```python
from build123d import *

# Parameters (mm, degrees)
BOSS_EXTRUDE1_DEPTH = 5
SKETCH2_W           = 12
SKETCH2_H           = 32
BOSS_EXTRUDE2_DEPTH = 6
CUT_EXTRUDE1_REACH  = 53.952
AGUJEROSMOTOR_R     = 1.5
FILLET1_R           = 2
SKETCH5_W           = 35
SKETCH5_H           = 5
BOSS_EXTRUDE3_DEPTH = 13
FILLET2_R           = 2
FILLET3_R           = 2
FILLET4_R           = 2
BOSS_EXTRUDE4_DEPTH = 3


with BuildPart() as part:
    # Sketch U → Boss-Extrude1 (new body)
    with BuildSketch(Plane(origin=(0, 0, 0), x_dir=(0, 0, -1), z_dir=(1, 0, 0))):
        with BuildLine():
            Line((0, 22), (0, 27))
            Line((0, 27), (-41, 27))
            ThreePointArc((-41, 27), (-42.414213562, 26.414213562), (-43, 25))
            Line((-43, 25), (-43, -3))
            ThreePointArc((-43, -3), (-42.414213562, -4.414213562), (-41, -5))
            Line((-41, -5), (0, -5))
            Line((0, -5), (0, 0))
            Line((0, 0), (-35, 0))
            ThreePointArc((-35, 0), (-36.414213562, 0.585786438), (-37, 2))
            Line((-37, 2), (-37, 20))
            ThreePointArc((-37, 20), (-36.414213562, 21.414213562), (-35, 22))
            Line((-35, 22), (0, 22))
        make_face()
    extrude(amount=-BOSS_EXTRUDE1_DEPTH)

    # Sketch2 → Boss-Extrude2 (add)
    with BuildSketch(Plane(origin=(0, 0, 0), x_dir=(0, 0, -1), z_dir=(1, 0, 0))):
        with Locations((-6, 11)):
            Rectangle(SKETCH2_W, SKETCH2_H)
    extrude(amount=BOSS_EXTRUDE2_DEPTH)

    # AgujerosMotor → Cut-Extrude1 (cut, up to next)
    with BuildSketch(Plane(origin=(6, 0, 0), x_dir=(0, 0, -1), z_dir=(1, 0, 0)), mode=Mode.PRIVATE) as cut_extrude1_sk1:
        with Locations((-5, 2)):
            Circle(AGUJEROSMOTOR_R)
    cut_extrude1_tool1 = extrude(cut_extrude1_sk1.sketch, amount=-CUT_EXTRUDE1_REACH, mode=Mode.PRIVATE) & part.part
    # AgujerosMotor → Cut-Extrude1 (cut, up to next)
    with BuildSketch(Plane(origin=(6, 0, 0), x_dir=(0, 0, -1), z_dir=(1, 0, 0)), mode=Mode.PRIVATE) as cut_extrude1_sk2:
        with Locations((-5, 20)):
            Circle(AGUJEROSMOTOR_R)
    cut_extrude1_tool2 = extrude(cut_extrude1_sk2.sketch, amount=-CUT_EXTRUDE1_REACH, mode=Mode.PRIVATE) & part.part
    add(cut_extrude1_tool1.solids().sort_by_distance((6, 2, 5))[0], mode=Mode.SUBTRACT)
    add(cut_extrude1_tool2.solids().sort_by_distance((6, 20, 5))[0], mode=Mode.SUBTRACT)

    # Fillet1
    fillet1_edges = [part.edges().sort_by_distance(p)[0] for p in [
        (6, 27, 6),
        (6, -5, 6),
    ]]
    fillet(fillet1_edges, radius=FILLET1_R)

    # Sketch5 → Boss-Extrude3 (add)
    with BuildSketch(Plane.ZY.offset(5)):
        with Locations((17.5, 24.5)):
            Rectangle(SKETCH5_W, SKETCH5_H)
    extrude(amount=BOSS_EXTRUDE3_DEPTH)

    # Fillet2
    fillet2_edges = [part.edges().sort_by_distance(p)[0] for p in [
        (-18, 24.5, 35),
    ]]
    fillet(fillet2_edges, radius=FILLET2_R)

    # Fillet3
    fillet3_edges = [part.edges().sort_by_distance(p)[0] for p in [
        (0, -5, 26.5),
        (0, -4.414213562, 42.414213562),
        (0, 11, 43),
        (0, 26.414213562, 42.414213562),
        (0, 27, 26.5),
        (-5, 26.414213562, 42.414213562),
        (-5, 11, 43),
        (-5, -4.414213562, 42.414213562),
        (-5, -5, 20.5),
        (6, 11, 12),
        (2, -5, 12),
        (2, 27, 12),
        (5.414213562, -4.414213562, 12),
        (5.414213562, 26.414213562, 12),
        (-5, 27, 38),
    ]]
    fillet(fillet3_edges, radius=FILLET3_R)

    # Fillet4
    fillet4_edges = [part.edges().sort_by_distance(p)[0] for p in [
        (-18, 27, 16.5),
        (-17.414213562, 27, 34.414213562),
        (-9.5, 27, 35),
    ]]
    fillet(fillet4_edges, radius=FILLET4_R)

    # Encastre → Boss-Extrude4 (add)
    with BuildSketch(Plane(origin=(0, 27, 0), x_dir=(1, 0, 0), z_dir=(0, 1, 0))):
        with BuildLine():
            Line((-5, -5), (-5, -25))
            ThreePointArc((-5, -25), (-9, -29), (-13, -25))
            Line((-13, -25), (-13, -5))
            ThreePointArc((-13, -5), (-9, -1), (-5, -5))
        make_face()
    extrude(amount=BOSS_EXTRUDE4_DEPTH)


solid = part.part
```
The model under review builds one solid part; all positions refer to its coordinate system, in mm. A direction names the side the tool comes from. Give positions to 0.01 mm unless a question says otherwise; leave off trailing zeros. Write each loop counter-clockwise with the first axis right and the second up, starting at its lowest first coordinate (ties: lowest second). Pieces come first, ordered by that corner, then holes. Notation, with made-up numbers: (72, 58) -> (100, 58) arc R17 ccw to (100, 63) -> close; hole circle Ø6 at (86, 1.5). An arc over 180 degrees is marked (long way). Answer in a Markdown table with one row per item.
1) Tool access review of faces 1 (the flat face through (0, 11, 6)), 2 (the cylindrical face through (-2.46, 0.57, 36.4)), 3 (the flat face through (-5, 28, 15)), 4 (the cylindrical face through (-9.41, 26.4, 34.43)): name each direction out of +Z, -Z, +X, -X, +Y, -Y from which nothing blocks a thin tool from reaching the whole face with its end or side.
Worked answers:
| item | result |
|---|---|
| face 1 | -Z, -X |
| face 2 | -Z, +X, -X |
| face 3 | +Z, -Z, +X, +Y |
| face 4 | +Z, -X, +Y |
2) Add section D-D on z = 23. State the section outline as (x, y) points, plus the area to 3 significant figures.
Worked answers:
| item | result |
|---|---|
| outline | (-18, 22) -> (0, 22) -> (0, 25) arc R2 ccw to (-2, 27) -> (-5, 27) -> (-5, 30) -> (-13, 30) -> (-13, 27) -> (-16, 27) arc R2 ccw to (-18, 25) -> close; (-5, -3) arc R2 ccw to (-3, -5) -> (-2, -5) arc R2 ccw to (0, -3) -> (0, 0) -> (-5, 0) -> close |
| area | 136 mm² |
3) Add section A-A on z = 32.5. State the section outline as (x, y) points, plus the area to 3 significant figures.
Worked answers:
| item | result |
|---|---|
| outline | (-18, 22) -> (0, 22) -> (0, 25) arc R2 ccw to (-2, 27) -> (-16, 27) arc R2 ccw to (-18, 25) -> close; (-5, -3) arc R2 ccw to (-3, -5) -> (-2, -5) arc R2 ccw to (0, -3) -> (0, 0) -> (-5, 0) -> close |
| area | 112 mm² |
4) For L1, parallel to Y at x = 2.6, z = 5; L2, parallel to Y at x = 4.55, z = 5; L3, parallel to Y at x = -9.5, z = 32.5, list the stretches that pass through material, from the lowest coordinate up. Write a range as [from, to].
Worked answers:
| item | result |
|---|---|
| L1 | [-5, 0.5], [3.5, 18.5], [21.5, 27] |
| L2 | [-4.92, 0.5], [3.5, 18.5], [21.5, 26.92] |
| L3 | [22, 27] |
5) Add section B-B on y = 16. State the section outline as (x, z) points.
Worked answers:
| item | result |
|---|---|
| outline | (-5, 37) -> (0, 37) -> (0, 41) arc R2 ccw to (-2, 43) -> (-3, 43) arc R2 ccw to (-5, 41) -> close; (0, 0) -> (6, 0) -> (6, 10) arc R2 ccw to (4, 12) -> (0, 12) -> close |
6) Add section C-C on x = -9. State the section outline as (y, z) points.
Worked answers:
| item | result |
|---|---|
| outline | (22, 0) -> (27, 0) -> (27, 1) -> (30, 1) -> (30, 29) -> (27, 29) -> (27, 33) arc R2 ccw to (25, 35) -> (22, 35) -> close |
7) Clearance check with flat-ended pins moving along their axes: P1, Ø3, axis at x = 3, y = 11.5, coming from the +Z side; P2, Ø14, axis at y = 10, z = 26.5, coming from the -X side; P3, Ø12, axis at y = 1.5, z = 29.5, coming from the +X side; P4, Ø4.5, axis at x = 2, y = 10, coming from the +Z side. State where each tip first meets the part, or that it passes through.
Worked answers:
| item | result |
|---|---|
| P1 | z = 12 |
| P2 | through |
| P3 | x = 0 |
| P4 | z = 41.97 |
